```python
from build123d import *

# Parameters (mm, degrees)
BOSS_EXTRUDE1_DEPTH  = 6.6
SKETCH4_W            = 6.6
SKETCH4_H            = 4.006069052
BOSS_EXTRUDE2_DEPTH  = 11
M4_CLEARANCE_HOLE1_D = 4.5


with BuildPart() as part:
    # Sketch2 → Boss-Extrude1 (new body)
    with BuildSketch(Plane.XY):
        Polygon((-48.677836014, 4.833253272), (-48.677836014, -6.166746728), (-78.677836014, -6.166746728), align=None)
    extrude(amount=BOSS_EXTRUDE1_DEPTH)

    # Sketch4 → Boss-Extrude2 (add)
    with BuildSketch(Plane(origin=(-48.677836014, 0, 0), x_dir=(0, 0, -1), z_dir=(1, 0, 0))):
        with Locations((-3.3, -4.163712202)):
            Rectangle(SKETCH4_W, SKETCH4_H)
    extrude(amount=BOSS_EXTRUDE2_DEPTH)

    # M4 Clearance Hole1 (through all)
    with Locations(Plane(origin=(-41.677836014, -2.160677676, 3.3), x_dir=(0, 0, 1), z_dir=(0, 1, 0))):
        with Locations((0, 0)):
            Hole(M4_CLEARANCE_HOLE1_D / 2)


solid = part.part
```
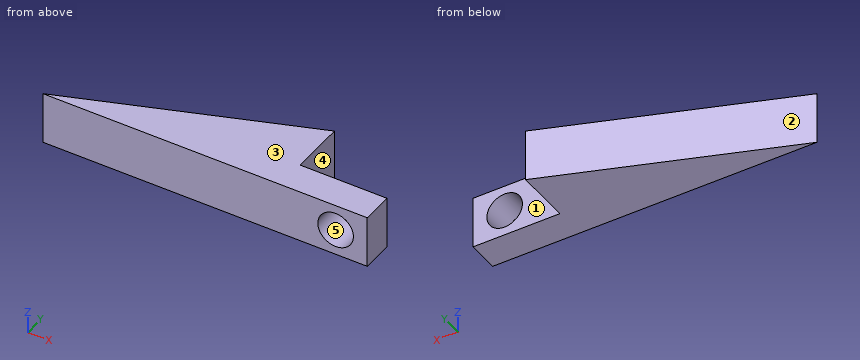
Geometry check sheet. Reference: the model listing, model coordinates, mm. Face numbers are marked on the shaded views. A direction names the side the tool comes from. Give positions to 0.01 mm unless a question says otherwise; leave off trailing zeros. Order: outer loops, then holes, each group sorted by start corner. A loop starts at its lowest first (then second) coordinate and runs counter-clockwise, first axis right, second up.
1. Section check C-C, the plane x = -71.5. Enter the section's corners in (y, z), and give its area (3 significant figures).
2. Thickness scan on L1, parallel to Y at x = -43.5, z = 5.5; L2, parallel to Y at x = -60.5, z = 1.5. Record the ranges inside material, lowest first.
3. Release check for a two-part mould opening along Z. For the marked faces 3, 4 and 5 record: pulls with the +Z half, pulls with the -Z half, needs draft (parallel to the pull), parting line crosses it, or undercut.
4. Section check D-D, the plane y = 3.5. Enter the section's corners in (x, z), and give its area (3 significant figures).
5. Gauge pin test, flat ends, axial feed: pin 1 Ø2 at (y, z) = (3, 1.5) entering from +X; pin 2 Ø2 at (x, z) = (-43.5, 4) entering from +Y; pin 3 Ø2 at (x, z) = (-68.5, 2) entering from +Y. Record the tip position at first contact, or that the pin passes through.
6. Section check A-A, the plane z = 3.3. Enter the section's corners in (x, y), and give its area (3 significant figures).
7. Section check B-B, the plane y = -5.25. Enter the section's corners in (x, z).
8. Access from +Z, -Z, +X, -X, +Y, -Y to the whole of each face (thin tool, end or side, straight path). Record for the marked faces 1 and 2.
Values follow:
1. outline: (-6.17, 0) - (-3.53, 0) - (-3.53, 6.6) - (-6.17, 6.6) - close
1. area: 17.4 mm2
2. L1: y = -6.17 to -2.16
2. L2: y = -6.17 to 0.5
3. face 3: pulls with the +Z half
3. face 4: needs draft
3. face 5: undercut
4. outline: (-52.31, 0) - (-48.68, 0) - (-48.68, 6.6) - (-52.31, 6.6) - close
4. area: 24.0 mm2
5. pin 1: stops at x = -48.68
5. pin 2: stops at y = -2.16
5. pin 3: stops at y = -2.07
6. outline: (-78.68, -6.17) - (-43.93, -6.17) - (-43.93, -2.16) - (-48.68, -2.16) - (-48.68, 4.83) - close; (-39.43, -6.17) - (-37.68, -6.17) - (-37.68, -2.16) - (-39.43, -2.16) - close
6. area: 191 mm2
7. outline: (-76.18, 0) - (-37.68, 0) - (-37.68, 6.6) - (-76.18, 6.6) - close; hole circle Ø4.5 at (-41.68, 3.3)
8. face 1: +Z, -Z, +X, +Y
8. face 2: +Z, -Z, -X, +Y
